Verification items for the finished model (mm, model axes). Coordinates: 2 decimals unless noted, no trailing zeros. Loops run counter-clockwise (first coordinate to the right, second up) from the corner with the lowest first, then second, coordinate; pieces in that order, holes last.
Q1. Sectioned sample at B-B (y = 4.25). Enter the section's corners in (x, z).
Q2. Material ranges on probe 1 along X at (y, z) = (5.5, 85); probe 2 along X at (y, z) = (4.25, 55); probe 3 along X at (y, z) = (6.25, 115), recorded low to high.
Q3. Sectioned sample at D-D (z = 79.5). Enter the section's corners in (x, y).
Q4. Sectioned sample at C-C (z = 116). Enter the section's corners in (x, y).
Q5. Go/stop test with flat-tipped pins: P1, Ø1, axis at y = 6, z = 92, coming from the +X side; P2, Ø4, axis at x = 85, z = 85, coming from the +Y side; P3, Ø4, axis at x = 59.5, y = 3, coming from the -Z side; P4, Ø1, axis at y = 7.5, z = 80.5, coming from the -X side. Record where each tip stops, or that it passes through.
Q6. Sectioned sample at A-A (x = 115). Enter the section's corners in (y, z).
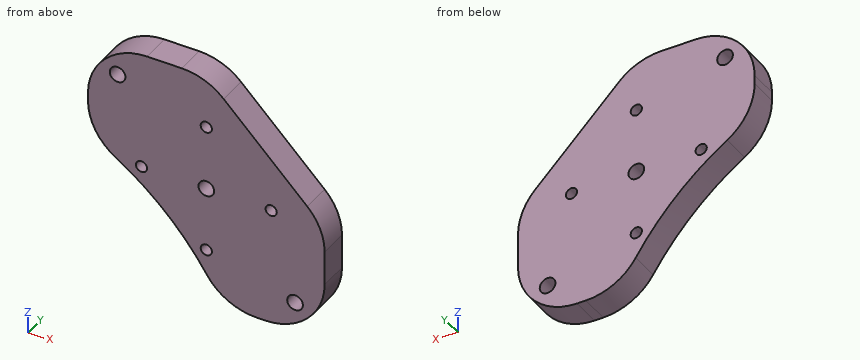
```python
from build123d import *

# Parameters (mm, degrees)
EXTRUDE_4_OUTLINE_R   = 2.65
EXTRUDE_4_OUTLINE_R_2 = 1.9
EXTRUDE_4_DEPTH       = 10
FILLET_2_R            = 20


# Read off the part's stored shape, not the designer's step: 凸台-拉伸4
with BuildPart() as part:
    # 凸台-拉伸4 outline → 凸台-拉伸4 (new body)
    with BuildSketch(Plane(origin=(0, 0, 0), x_dir=(1, 0, 0), z_dir=(0, 1, 0))):
        with BuildLine():
            Line((85, -125), (125, -85))
            Line((125, -85), (125, -45))
            Line((125, -45), (90.421236444, -45))
            ThreePointArc((90.421236444, -45), (71.4177849, -71.4177849), (45, -90.421236444))
            Line((45, -90.421236444), (45, -125))
            Line((45, -125), (85, -125))
        make_face()
        with Locations((55, -115)):
            Circle(EXTRUDE_4_OUTLINE_R, mode=Mode.SUBTRACT)
        with Locations((85, -106.920310217)):
            Circle(EXTRUDE_4_OUTLINE_R_2, mode=Mode.SUBTRACT)
        with Locations((63.079689783, -85)):
            Circle(EXTRUDE_4_OUTLINE_R_2, mode=Mode.SUBTRACT)
        with Locations((85, -85)):
            Circle(EXTRUDE_4_OUTLINE_R, mode=Mode.SUBTRACT)
        with Locations((106.920310217, -85)):
            Circle(EXTRUDE_4_OUTLINE_R_2, mode=Mode.SUBTRACT)
        with Locations((85, -63.079689783)):
            Circle(EXTRUDE_4_OUTLINE_R_2, mode=Mode.SUBTRACT)
        with Locations((115, -55)):
            Circle(EXTRUDE_4_OUTLINE_R, mode=Mode.SUBTRACT)
    extrude(amount=EXTRUDE_4_DEPTH)

    # 圆角2
    fillet_2_edges = [part.edges().sort_by_distance(p)[0] for p in [
        (85, 5, 125),
        (45, 5, 125),
        (45, 5, 90.421236444),
        (90.421236444, 5, 45),
        (125, 5, 45),
        (125, 5, 85),
    ]]
    fillet(fillet_2_edges, radius=FILLET_2_R)


solid = part.part
```
Geometry check:
1. outline: (45, 102.06) arc R20 ccw to (54.26, 85.19) arc R101 cw to (85.19, 54.26) arc R20 ccw to (102.06, 45) - (105, 45) arc R20 ccw to (125, 65) - (125, 76.72) arc R20 ccw to (119.14, 90.86) - (90.86, 119.14) arc R20 ccw to (76.72, 125) - (65, 125) arc R20 ccw to (45, 105) - close; hole circle Ø5.3 at (55, 115); hole circle Ø3.8 at (63.08, 85); hole circle Ø5.3 at (85, 85); hole circle Ø3.8 at (85, 63.08); hole circle Ø3.8 at (85, 106.92); hole circle Ø3.8 at (106.92, 85); hole circle Ø5.3 at (115, 55)
2. probe 1: x = 54.55 to 61.18, 64.98 to 82.35, 87.65 to 105.02, 108.82 to 123.2
2. probe 2: x = 84.71 to 112.35, 117.65 to 122.32
2. probe 3: x = 47.68 to 52.35, 57.65 to 95
3. outline: (62.3, 0) - (124.81, 0) - (124.81, 10) - (62.3, 10) - close
4. outline: (48.3, 0) - (52.55, 0) - (52.55, 10) - (48.3, 10) - close; (57.45, 0) - (94, 0) - (94, 10) - (57.45, 10) - close
5. P1: stops at x = 118.5
5. P2: passes through
5. P3: stops at z = 80.12
5. P4: stops at x = 60.33
6. outline: (0, 47.68) - (10, 47.68) - (10, 52.35) - (0, 52.35) - close; (0, 57.65) - (10, 57.65) - (10, 95) - (0, 95) - close
